```python
from build123d import *

# Parameters (mm, degrees)
F0_R            = 44.8437
F0_R_2          = 17.4625
F0_W            = 19.05
F0_H            = 6.35
F1_DEPTH        = 12.7
F2_DEPTH        = 6.35
F2_COPIES_COUNT = 4
F3_DEPTH        = 12.701
F3_COPIES_COUNT = 4
F5_DEPTH        = 25.4


# Not quite as in the source:
# - a pattern or mirror of a feature is missing from the dataset's text; its kind, count and spacing are read off the source's solid


with BuildPart() as f1:
    # F0 (on Top) → F1 (new body)
    with BuildSketch(Plane.XY):
        with BuildLine():
            ThreePointArc((-9.525, 139.3749058296), (-95.3557746023, -102.0948884617), (139.7, 0))
            ThreePointArc((139.7, 0), (102.0948884617, 95.3557746023), (9.525, 139.3749058296))
            Line((9.525, 139.3749058296), (9.525, 120.3249058296))
            Line((9.525, 120.3249058296), (9.525, 113.9749058296))
            Line((9.525, 113.9749058296), (-9.525, 113.9749058296))
            Line((-9.525, 113.9749058296), (-9.525, 120.3249058296))
            Line((-9.525, 120.3249058296), (-9.525, 139.3749058296))
        make_face()
        Circle(F0_R, mode=Mode.SUBTRACT)
        with Locations((101.4398184138, 36.921074472)):
            Circle(F0_R_2, mode=Mode.SUBTRACT)
        with Locations((36.921074472, 101.4398184138)):
            Circle(F0_R_2, mode=Mode.SUBTRACT)
        with Locations((76.3321770291, 76.3321770291)):
            Circle(F0_R_2, mode=Mode.SUBTRACT)
        with BuildLine():
            Line((9.525, 120.3249058296), (9.525, 139.3749058296))
            ThreePointArc((9.525, 139.3749058296), (0, 139.7), (-9.525, 139.3749058296))
            Line((-9.525, 139.3749058296), (-9.525, 120.3249058296))
            Line((-9.525, 120.3249058296), (9.525, 120.3249058296))
        make_face()
        with Locations((36.921074472, 101.4398184138)):
            Circle(F0_R_2)
        with Locations((76.3321770291, 76.3321770291)):
            Circle(F0_R_2)
        with Locations((101.4398184138, 36.921074472)):
            Circle(F0_R_2)
        with Locations((0, 117.1499058296)):
            Rectangle(F0_W, F0_H)
        Circle(F0_R)
    extrude(amount=-F1_DEPTH)

    # F0 (on Top) → F2 (cut)
    with BuildSketch(Plane.XY):
        with Locations((36.921074472, 101.4398184138)):
            Circle(F0_R_2)
        with Locations((76.3321770291, 76.3321770291)):
            Circle(F0_R_2)
        with Locations((101.4398184138, 36.921074472)):
            Circle(F0_R_2)
    f2 = extrude(amount=-F2_DEPTH, mode=Mode.SUBTRACT)

    # F2_copies: F2 ×4 about axis
    f2_copies_axis = Axis((0, 0, 0), (0, 0, 1))
    for i in range(1, F2_COPIES_COUNT):
        add(f2.rotate(f2_copies_axis, i * 360 / F2_COPIES_COUNT), mode=Mode.SUBTRACT)

    # F0 (on Top) → F3 (cut, through all)
    with BuildSketch(Plane.XY):
        with BuildLine():
            Line((9.525, 120.3249058296), (9.525, 139.3749058296))
            ThreePointArc((9.525, 139.3749058296), (0, 139.7), (-9.525, 139.3749058296))
            Line((-9.525, 139.3749058296), (-9.525, 120.3249058296))
            Line((-9.525, 120.3249058296), (9.525, 120.3249058296))
        make_face()
    f3 = extrude(amount=-F3_DEPTH, mode=Mode.SUBTRACT)

    # F3_copies: F3 ×4 about axis
    f3_copies_axis = Axis((0, 0, 0), (0, 0, 1))
    for i in range(1, F3_COPIES_COUNT):
        add(f3.rotate(f3_copies_axis, i * 360 / F3_COPIES_COUNT), mode=Mode.SUBTRACT)

    # F0 (on Top) → F5 (cut)
    with BuildSketch(Plane.XY):
        Circle(F0_R)
    extrude(amount=-F5_DEPTH, mode=Mode.SUBTRACT)


solid = f1.part
```
Input: part model. Units: mm. Frame: model coordinates. A direction names the side the tool comes from. Round coordinates to 2 decimals unless told otherwise and drop trailing zeros. Order: outer loops, then holes, each group sorted by start corner. A loop starts at its lowest first (then second) coordinate and runs counter-clockwise, first axis right, second up. Notation, with made-up numbers: (3.25, -8) - (14.25, -8) arc R26 ccw to (14.25, 19) - close; hole circle Ø6 at (66, 1). An arc over 180 degrees is marked (long way). One line per question, with ' | ' between items. Start each with the question number.
1) Cut plane C-C, the plane z = -10.75. Return the cut outline in (x, y) (3 decimals), then the cut area to 3 significant figures.
2) Cut plane D-D, the plane y = -115. Return the cut outline in (x, z).
3) Cut plane A-A, the plane x = 0. Return the cut outline in (y, z).
4) Contact query for flat-ended pins moving along their axis: P1, Ø2, axis at x = -48, z = -5, coming from the -Y side; P2, Ø2, axis at y = -34, z = -3, coming from the -X side; P3, Ø2, axis at x = 94, z = -3, coming from the -Y side. Output: stop coordinate, or through.
5) Set-up query: faces 1 (the cylindrical face through (81.577, -92.988, -3.131)), 2 (the flat face through (120.325, 0, -6)), 3 (the flat face through (0, 120.325, -6)). Return all of +Z, -Z, +X, -X, +Y, -Y with unobstructed straight access to the full face (end or side cutting, diameter ignored); none if empty.
6) Ray query, probe 1 along X at (y, z) = (75, -4.5); probe 2 along X at (y, z) = (61.5, -6.25); probe 3 along Y at (x, z) = (48, -2.5). Return the intervals inside material, ascending.
7) Pull-direction query (X, two-part tool) for faces 4 (the flat face through (-33, 33, 0)), 5 (the cylindrical face through (99.77, 97.786, -6.261)), 6 (the cylindrical face through (92.988, 81.577, -3.131)); classes: +X half, -X half, draft (parallel to the pull), parting line (faces both ways), or undercut.
Worked out:
1) outline: (-139.375, -9.525) arc R139.7 ccw to (-9.525, -139.375) - (-9.525, -120.325) - (9.525, -120.325) - (9.525, -139.375) arc R139.7 ccw to (139.375, -9.525) - (120.325, -9.525) - (120.325, 9.525) - (139.375, 9.525) arc R139.7 ccw to (9.525, 139.375) - (9.525, 120.325) - (-9.525, 120.325) - (-9.525, 139.375) arc R139.7 ccw to (-139.375, 9.525) - (-120.325, 9.525) - (-120.325, -9.525) - close; hole circle Ø89.687 at (0, 0) | area: 53,500 mm^2
2) outline: (-79.32, -12.7) - (79.32, -12.7) - (79.32, 0) - (47.92, 0) - (47.92, -6.35) - (25.92, -6.35) - (25.92, 0) - (-25.92, 0) - (-25.92, -6.35) - (-47.92, -6.35) - (-47.92, 0) - (-79.32, 0) - close
3) outline: (-120.32, -12.7) - (-44.84, -12.7) - (-44.84, 0) - (-120.32, 0) - close; (44.84, -12.7) - (120.32, -12.7) - (120.32, 0) - (44.84, 0) - close
4) P1: stops at y = -131.56 | P2: stops at x = -135.75 | P3: stops at y = -104.25
5) face 1: +Z | face 2: +Z, -Z, +X | face 3: +Z, -Z, +Y
6) probe 1: x = -117.86 to -93.74, -58.92 to 58.92, 93.74 to 117.86 | probe 2: x = -125.43 to -85.55, -67.12 to 67.12, 85.55 to 125.43 | probe 3: y = -131.19 to -114.94, -87.94 to 87.94, 114.94 to 131.19
7) face 4: draft | face 5: +X half | face 6: undercut
